Input: part model. Units: mm. Frame: model coordinates. A direction names the side the tool comes from. Round coordinates to 2 decimals unless told otherwise and drop trailing zeros. Write each loop counter-clockwise with the first axis right and the second up, starting at its lowest first coordinate (ties: lowest second). Pieces come first, ordered by that corner, then holes. Notation, with made-up numbers: (12.5, 63.25) - (67.5, 63.25) arc R30 ccw to (67.5, 99.25) - close; hole circle Ø5 at (88, 47.25). An arc over 180 degrees is marked (long way). One line per item, written item: value. Start each with the question number.
Autodesk Inventor part; units mm, degrees
ref_plane "YZ Plane" through (0, 0, 0) normal (1, 0, 0) x (0, 1, 0)
ref_plane "XZ Plane" through (0, 0, 0) normal (0, 1, 0) x (-1, 0, 0)
ref_plane "XY Plane" through (0, 0, 0) normal (0, 0, 1) x (1, 0, 0)
sketch "Sketch1" plane through (0, 0, 0) normal (1, 0, 0) x (0, 1, 0)
  line L0 (5.5, 10) -> (5.5, 10)
  line L1 (8.5, 0) -> (9, 0)
  line L2 (9, 0) -> (9, 10)
  line L3 (9, 10) -> (5.5, 10)
  line L4 (0, 0) -> (0, 4.238)
  line L5 (5.5, 10) -> (8.5, 0)
  dimension "d11" = 0
  dimension "d13" = 9
  dimension "d14" = 5.5
  dimension "d15" = 10
  dimension "d26" = 8.5
revolve "Revolution1" add sketch "Sketch1" angle 360 about axis through (0, 0, 0) along (0, 0, 1)
sketch "Sketch3" plane through (0, 0, 0) normal (0, 0, -1) x (-1, 0, 0)
  line L0 (-5.5, 0) -> (5.5, 0)
  line L1 (5.5, 0) -> (5.5, -9)
  line L2 (5.5, -9) -> (-5.5, -9)
  line L3 (-5.5, -9) -> (-5.5, 0)
  circle A0 centre (0, 0) radius 9
  circle A1 centre (0, 0) radius 5.5
extrude "Extrusion1" cut sketch "Sketch3" against normal blind 10 contours A1 L1 A0 L3 | L0 A1 | A0 L2 L3 | L1 L2 A0 picked at (4.148, -6.5999) picked at (-1.2514, -2.3608)
fillet "Fillet1" radius 1 5 edges at (0, 8.5, 0) (5.5, -6.8023, 0) (-5.5, -6.8023, 0) (-5.5, -7.1239, 5) (5.5, -7.1239, 5)
sketch "Sketch4" plane through (0, 0, 10) normal (0, 0, 1) x (1, 0, 0)
  line L0 (-5, 17.4833) -> (5, 17.4833)
  line L1 (5, 17.4833) -> (5, 7.4833)
  line L2 (5, 7.4833) -> (-5, 7.4833)
  line L3 (-5, 7.4833) -> (-5, 17.4833)
  circle A0 centre (0, 13.0699) radius 1.6
  arc A1 (7.3125, -5.2467) -> (-7.3125, -5.2467) centre (0, 0) ccw
  dimension "d19" = 10
  dimension "d21" = 10
  dimension "d22" = 3.2
  dimension "d29" = 4.4135
extrude "Extrusion2" add sketch "Sketch4" against normal blind 5 contours L0 L1 A1 L3
fillet "Fillet2" radius 2 2 edges at (5, 17.4833, 7.5) (-5, 17.4833, 7.5)
properties part number "brush rack"
Q1. Cut plane A-A, the plane x = 0. Output: boundary loops of the cut face in (y, z).
Q2. Cut plane C-C, the plane z = 3. Output: boundary loops of the cut face in (x, y), and give its area (3 significant figures).
Q3. Material intervals for probe 1 along X at (y, z) = (15, 9.5); probe 2 along Y at (x, z) = (0, 7.3); probe 3 along X at (y, z) = (-4.5, 5.75), sorted ascending. Write a range as from..to.
Q4. Cut plane D-D, the plane z = 7.5. Output: boundary loops of the cut face in (x, y), and give its area (3 significant figures).
Q5. Cut plane B-B, the plane z = 5.5. Output: boundary loops of the cut face in (x, y), and give its area (3 significant figures).
Q6. Contact query for flat-ended pins moving along their axis: pin 1 Ø1.5 at (y, z) = (1.5, 5) entering from +X; pin 2 Ø2.5 at (y, z) = (-2.5, 6.5) entering from +X; pin 3 Ø2 at (y, z) = (6.5, 8) entering from -X. Output: stop coordinate, or through.
Q7. Access query for faces 1 (the cylindrical face through (0, 9, 4)), 2 (the flat face through (-5.5, -4, 8)), 3 (the flat face through (-5, 11, 8)). Directions: +Z, -Z, +X, -X, +Y, -Y. A direction counts if a zero-diameter tool reaches every point of the face in a straight line with its end or side. Return the directions, or none.
Q8. Pull-direction query (X, two-part tool) for faces 4 (the cylindrical face through (-4.43, 16.88, 7.46)), 5 (the flat face through (5.5, -3, 8)), 6 (the flat face through (0, 11, 5)); classes: pulls with the +X half, pulls with the -X half, needs draft (parallel to the pull), parting line crosses it, or undercut.
A:
1. outline: (5.5, 10) - (8.3, 0.68) arc R1 ccw to (9, 0) - (9, 5) - (11.47, 5) - (11.47, 10) - close; (14.67, 5) - (17.48, 5) - (17.48, 10) - (14.67, 10) - close
2. outline: (-7.31, -5.25) arc R1 ccw to (-5.61, -5.12) arc R7.6 cw (long way) to (5.61, -5.12) arc R1 ccw to (7.31, -5.25) arc R9 ccw (long way) to start
2. area: 53.4 mm²
3. probe 1: x = -5..5
3. probe 2: y = 6.31..11.47, 14.67..17.48
3. probe 3: x = -7.79..-5.5, 5.5..7.79
4. outline: (-7.31, -5.25) arc R1 ccw to (-5.5, -4.66) - (-5.5, -2.97) arc R6.25 cw (long way) to (5.5, -2.97) - (5.5, -4.66) arc R1 ccw to (7.31, -5.25) arc R9 ccw to (5, 7.48) - (5, 15.48) arc R2 ccw to (3, 17.48) - (-3, 17.48) arc R2 ccw to (-5, 15.48) - (-5, 7.48) arc R9 ccw to start; hole circle Ø3.2 at (0, 13.07)
4. area: 175 mm²
5. outline: (-7.31, -5.25) arc R1 ccw to (-5.5, -4.66) - (-5.5, -4.08) arc R6.85 cw (long way) to (5.5, -4.08) - (5.5, -4.66) arc R1 ccw to (7.31, -5.25) arc R9 ccw to (5, 7.48) - (5, 15.48) arc R2 ccw to (3, 17.48) - (-3, 17.48) arc R2 ccw to (-5, 15.48) - (-5, 7.48) arc R9 ccw to start; hole circle Ø3.2 at (0, 13.07)
5. area: 158 mm²
6. pin 1: stops at x = 8.97
6. pin 2: stops at x = 8.91
6. pin 3: stops at x = -7.12
7. face 1: -Z
7. face 2: +Z, -Z, -Y
7. face 3: +Z, -Z, -X, +Y
8. face 4: pulls with the -X half
8. face 5: undercut
8. face 6: needs draft
